```python
from build123d import *

# Parameters (mm, degrees)
BOSS_EXTRUDE1_DEPTH = 1.5875
SKETCH4_W           = 11.3
SKETCH4_H           = 63.35
SKETCH4_R           = 1.59
CUT_EXTRUDE2_DEPTH  = 3.175


with BuildPart() as part:
    # Sketch2 → Boss-Extrude1 (new body, symmetric)
    with BuildSketch(Plane(origin=(0, 0, 0), x_dir=(1, 0, 0), z_dir=(0, 1, 0))):
        Polygon((-50.03165, -32.99970686), (-52.06365, -32.99970686), (-52.06365, -45.96770686), (48.00035, -45.96770686), (48.00035, -32.99970686), (45.96835, -32.99970686), (45.96835, 33.00029314), (48.00035, 33.00029314), (48.00035, 45.96829314), (-52.06365, 45.96829314), (-52.06365, 33.00029314), (-50.03165, 33.00029314), align=None)
    extrude(amount=BOSS_EXTRUDE1_DEPTH, both=True)

    # Sketch4 → Cut-Extrude2 (cut)
    with BuildSketch(Plane(origin=(0, 1.5875, 0), x_dir=(1, 0, 0), z_dir=(0, 1, 0))):
        with Locations((-42.47165, 0.055)):
            Rectangle(SKETCH4_W, SKETCH4_H)
        with Locations((-44.95165, 37.465)):
            Circle(SKETCH4_R)
        Polygon((32.26835, -40.255), (37.21835, -40.255), (37.21835, -19.935), (42.29835, -19.935), (42.29835, 31.375), (37.21835, 31.375), (37.21835, 41.535), (32.26835, 41.535), align=None)
        with Locations((40.77835, -40.005)):
            Circle(SKETCH4_R)
        with Locations((40.77835, 40.005)):
            Circle(SKETCH4_R)
        with Locations((-44.95165, -36.195)):
            Circle(SKETCH4_R)
    extrude(amount=-CUT_EXTRUDE2_DEPTH, mode=Mode.SUBTRACT)


solid = part.part
```
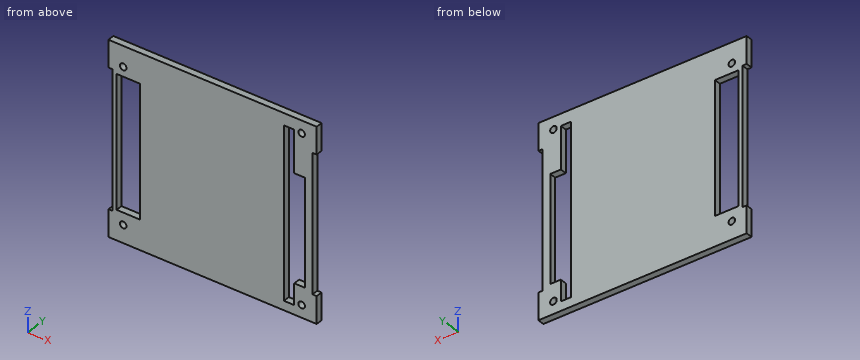
Input: part model. Units: mm. Frame: model coordinates. Give positions to 0.01 mm unless a question says otherwise; leave off trailing zeros. Order: outer loops, then holes, each group sorted by start corner. A loop starts at its lowest first (then second) coordinate and runs counter-clockwise, first axis right, second up. Notation, with made-up numbers: M 54.5,81.25 L 113.5,81.25 A26 ccw 113.5,102.25 Z; hole C -6.5,43.5 d3. An arc over 180 degrees is marked long. One line per question, with ' | ' between items.
1) Section A-A on z = 26.5. Output: boundary loops of the cut face in (x, y).
Filled in:
outline: M -50.03,-1.59 L -48.12,-1.59 L -48.12,1.59 L -50.03,1.59 Z; M -36.82,-1.59 L 32.27,-1.59 L 32.27,1.59 L -36.82,1.59 Z; M 37.22,-1.59 L 45.97,-1.59 L 45.97,1.59 L 37.22,1.59 Z
2) Ray query, L1, parallel to X at y = 0.7, z = 4; L2, parallel to Z at x = 34.5, y = 0.1 (3 decimals); L3, parallel to X at y = 0.55, z = 25. Return the intervals inside material, ascending.
Filled in:
L1: x = -50.03 to -48.12, -36.82 to 32.27, 42.3 to 45.97 | L2: z = -45.968 to -41.535, 40.255 to 45.968 | L3: x = -50.03 to -48.12, -36.82 to 32.27, 37.22 to 45.97
3) Contact query for flat-ended pins moving along their axis: P1, Ø1, axis at y = 0, z = 4, coming from the +X side; P2, Ø2.5, axis at x = -44.95, z = -37.47, coming from the -Y side; P3, Ø1.6, axis at y = 0, z = 31, coming from the -X side. Output: stop coordinate, or through.
Filled in:
P1: stops at x = 45.97 | P2: passes through | P3: stops at x = -50.03
4) Section B-B on z = 17. Output: boundary loops of the cut face in (x, y), and give its area (3 significant figures).
Filled in:
outline: M -50.03,-1.59 L -48.12,-1.59 L -48.12,1.59 L -50.03,1.59 Z; M -36.82,-1.59 L 32.27,-1.59 L 32.27,1.59 L -36.82,1.59 Z; M 42.3,-1.59 L 45.97,-1.59 L 45.97,1.59 L 42.3,1.59 Z | area: 237 mm2
5) Section C-C on y = -0.1. Output: boundary loops of the cut face in (x, z) (3 decimals).
Filled in:
outline: M -52.064,-45.968 L 48,-45.968 L 48,-33 L 45.968,-33 L 45.968,33 L 48,33 L 48,45.968 L -52.064,45.968 L -52.064,33 L -50.032,33 L -50.032,-33 L -52.064,-33 Z; hole M -48.122,-31.73 L -36.822,-31.73 L -36.822,31.62 L -48.122,31.62 Z; hole C -44.952,-37.465 d3.18; hole C -44.952,36.195 d3.18; hole M 32.268,-41.535 L 37.218,-41.535 L 37.218,-31.375 L 42.298,-31.375 L 42.298,19.935 L 37.218,19.935 L 37.218,40.255 L 32.268,40.255 Z; hole C 40.778,-40.005 d3.18; hole C 40.778,40.005 d3.18
